Geometry: final body of the model. Coordinates: model frame, mm. Give positions to 0.01 mm unless a question says otherwise; leave off trailing zeros. Order: outer loops, then holes, each group sorted by start corner. A loop starts at its lowest first (then second) coordinate and runs counter-clockwise, first axis right, second up. Notation, with made-up numbers: M 64.25,-12.5 L 84.25,-12.5 A15 cw 84.25,4.5 Z; hole C 52.5,16 d6. An arc over 180 degrees is marked long. One line per item, written item: value. Start each with the question number.
```python
from build123d import *

# Parameters (mm, degrees)
F0_R     = 2
F1_DEPTH = 5


with BuildPart() as f1:
    # F0 (on Front) → F1 (new body)
    with BuildSketch(Plane.XZ):
        with BuildLine():
            Line((0, 165), (0, 0))
            Line((0, 0), (95, 0))
            ThreePointArc((95, 0), (102.071068, 2.928932), (105, 10))
            Line((105, 10), (105, 155))
            ThreePointArc((105, 155), (102.071068, 162.071068), (95, 165))
            Line((95, 165), (0, 165))
        make_face()
        with BuildLine():
            ThreePointArc((89.5, 30), (86.085786, 28.585786), (87.5, 32))
            ThreePointArc((87.5, 32), (88.914214, 31.414214), (89.5, 30))
        make_face(mode=Mode.SUBTRACT)
        with Locations((30, 147.5)):
            Circle(F0_R, mode=Mode.SUBTRACT)
        with BuildLine():
            ThreePointArc((87.5, 118), (86.085786, 121.414214), (89.5, 120))
            ThreePointArc((89.5, 120), (88.914214, 118.585786), (87.5, 118))
        make_face(mode=Mode.SUBTRACT)
    extrude(amount=F1_DEPTH)


solid = f1.part
```
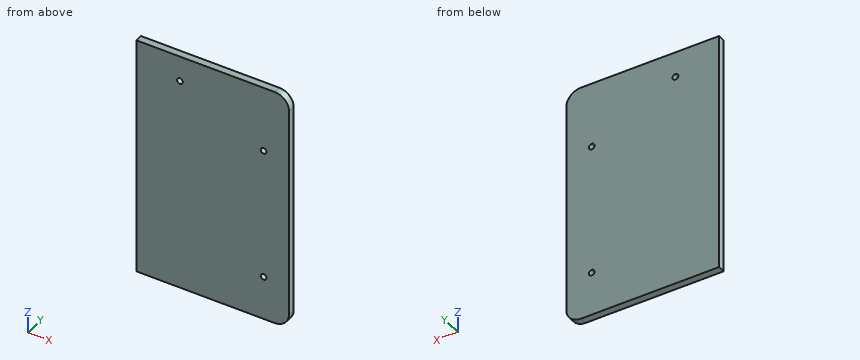
Q1. Section query A-A on z = 147.5. Return loops of the section in (x, y), and give its area (3 significant figures).
Q2. Section query B-B on x = 30. Return loops of the section in (y, z), and give its area (3 significant figures).
Q3. Ray query, line 1 along Z through (x, y) = (87.5, -4); line 2 along X through (y, z) = (-3.2, 147.5); line 3 along X through (y, z) = (-2.7, 30). Return the intervals inside material, ascending. Write a range as [from, to].
Results below:
1. outline: M 0,-5 L 28,-5 L 28,0 L 0,0 Z; M 32,-5 L 105,-5 L 105,0 L 32,0 Z
1. area: 505 mm2
2. outline: M -5,0 L 0,0 L 0,145.5 L -5,145.5 Z; M -5,149.5 L 0,149.5 L 0,165 L -5,165 Z
2. area: 805 mm2
3. line 1: [0, 28], [32, 118], [122, 165]
3. line 2: [0, 28], [32, 105]
3. line 3: [0, 85.5], [89.5, 105]
